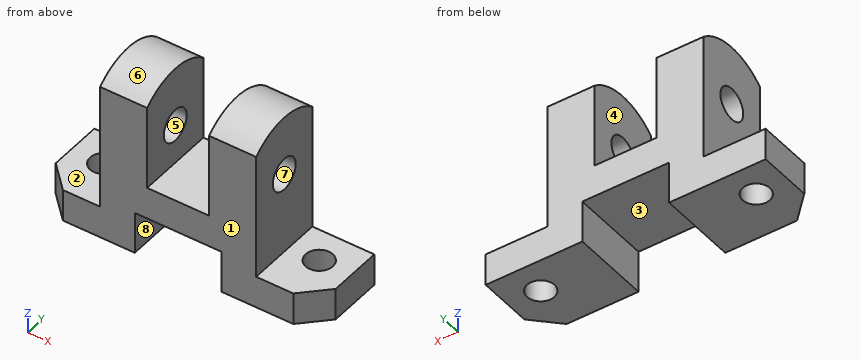
```python
from build123d import *

# Parameters (mm, degrees)
F1_DEPTH  = 32
F3_DEPTH  = 13.001
F5_DEPTH  = 13.001
F6_R      = 5.5
F7_DEPTH  = 13.001
F9_DEPTH  = 19
F11_DEPTH = 19
F13_R     = 6.5
F14_DEPTH = 100.001


with BuildPart() as f1:
    # F0 (on Front) → F1 (new body)
    with BuildSketch(Plane.XZ):
        Polygon((0, 13), (0, 0), (39, 0), (39, 17), (74, 17), (74, 0), (113, 0), (113, 13), (88, 13), (88, 64), (69, 64), (69, 30), (44, 30), (44, 64), (25, 64), (25, 13), align=None)
    extrude(amount=-F1_DEPTH)

    # F2 (on face) → F3 (cut, through all)
    with BuildSketch(Plane.XY.offset(13)):
        Polygon((113, 10), (103, 0), (113, 0), align=None)
    extrude(amount=-F3_DEPTH, mode=Mode.SUBTRACT)

    # F4 (on face) → F5 (cut, through all)
    with BuildSketch(Plane.XY.offset(13)):
        Polygon((0, 10), (0, 0), (10, 0), align=None)
    extrude(amount=-F5_DEPTH, mode=Mode.SUBTRACT)

    # F6 (on face) → F7 (cut, through all)
    with BuildSketch(Plane.XY.offset(13)):
        with Locations((13, 19)):
            Circle(F6_R)
        with Locations((100, 19)):
            Circle(F6_R)
    extrude(amount=-F7_DEPTH, mode=Mode.SUBTRACT)

    # F8 (on face) → F9 (join)
    with BuildSketch(Plane.YZ.offset(88)):
        with BuildLine():
            Line((0, 64), (32, 64))
            ThreePointArc((32, 64), (16, 70.083189), (0, 64))
        make_face()
    extrude(amount=-F9_DEPTH)

    # F10 (on face) → F11 (join)
    with BuildSketch(Plane(origin=(25, 0, 0), x_dir=(0, -1, 0), z_dir=(-1, 0, 0))):
        with BuildLine():
            Line((-32, 64), (0, 64))
            ThreePointArc((0, 64), (-16, 70.083189), (-32, 64))
        make_face()
    extrude(amount=-F11_DEPTH)

    # F13 (on offset) → F14 (cut, through all)
    with BuildSketch(Plane.YZ.offset(100)):
        with Locations((16, 46)):
            Circle(F13_R)
    extrude(amount=-F14_DEPTH, mode=Mode.SUBTRACT)


solid = f1.part
```
For this review, take the finished solid that the model builds, in its own axes (mm). Face numbers are marked on the shaded views. A direction names the side the tool comes from. Round coordinates to 2 decimals unless told otherwise and drop trailing zeros. Write each loop counter-clockwise with the first axis right and the second up, starting at its lowest first coordinate (ties: lowest second). Pieces come first, ordered by that corner, then holes. Notation, with made-up numbers: (51.5, 5) - (69.5, 5) arc R15 cw to (69.5, 25) - close; hole circle Ø3 at (17, -16.5). An arc over 180 degrees is marked (long way). Answer as a JSON object with one key per item and string values.
1. We need section B-B on x = 13. Give the boundary of the cut face in (y, z), then the cut area to 3 significant figures.
Response values:
{"outline": "(0, 0) - (13.5, 0) - (13.5, 13) - (0, 13) - close; (24.5, 0) - (32, 0) - (32, 13) - (24.5, 13) - close", "area": "273 mm2"}
2. Tool access review of the marked faces 1, 2, 3 and 4: name each direction out of +Z, -Z, +X, -X, +Y, -Y from which nothing blocks a thin tool from reaching the whole face with its end or side.
Response values:
{"face 1": "+Z, -Z, +X, -X, -Y", "face 2": "+Z, -X, +Y, -Y", "face 3": "-Z, +Y, -Y", "face 4": "+Z, +Y, -Y"}
3. We need section A-A on z = 11. Give the boundary of the cut face in (x, y).
Response values:
{"outline": "(0, 10) - (10, 0) - (39, 0) - (39, 32) - (0, 32) - close; (74, 0) - (103, 0) - (113, 10) - (113, 32) - (74, 32) - close; hole circle Ø11 at (13, 19); hole circle Ø11 at (100, 19)"}
4. We need section D-D on z = 46. Give the boundary of the cut face in (x, y), then the cut area to 3 significant figures.
Response values:
{"outline": "(25, 0) - (44, 0) - (44, 9.5) - (25, 9.5) - close; (25, 22.5) - (44, 22.5) - (44, 32) - (25, 32) - close; (69, 0) - (88, 0) - (88, 9.5) - (69, 9.5) - close; (69, 22.5) - (88, 22.5) - (88, 32) - (69, 32) - close", "area": "722 mm2"}
5. We need section C-C on z = 32. Give the boundary of the cut face in (x, y).
Response values:
{"outline": "(25, 0) - (44, 0) - (44, 32) - (25, 32) - close; (69, 0) - (88, 0) - (88, 32) - (69, 32) - close"}
6. Draft analysis for pull direction Z (two halves, no side actions). For the marked faces 5, 6, 7 and 8, state which applies: +Z half, -Z half, draft (parallel to the pull), parting line (faces both ways), or undercut.
Response values:
{"face 5": "undercut", "face 6": "+Z half", "face 7": "undercut", "face 8": "draft"}
7. To check wall thickness, follow line 1 along X through (y, z) = (19.5, 6); line 2 along X through (y, z) = (12, 5.5); line 3 along Z through (x, y) = (38.5, 16). State the ranges of each line that lie inside material, in increasing order.
Response values:
{"line 1": "x = 0 to 7.52, 18.48 to 39, 74 to 94.52, 105.48 to 113", "line 2": "x = 0 to 39, 74 to 113", "line 3": "z = 0 to 39.5, 52.5 to 70.08"}
8. For pin 1 Ø1.5 at (x, y) = (55.5, 19.5) entering from +Z; pin 2 Ø10 at (y, z) = (9.5, 50) entering from -X; pin 3 Ø9.5 at (y, z) = (10, 43.5) entering from +X; pin 4 Ø11.5 at (y, z) = (16, 46) entering from +X, all flat-tipped, find the tip position at first contact; note any pin that passes through.
Response values:
{"pin 1": "stops at z = 30", "pin 2": "stops at x = 25", "pin 3": "stops at x = 88", "pin 4": "passes through"}
